Source: CAD feature listing. Evaluate the final solid. Frame: model axes, mm. A direction names the side the tool comes from. Give positions to 0.01 mm unless a question says otherwise; leave off trailing zeros. Write each loop counter-clockwise with the first axis right and the second up, starting at its lowest first coordinate (ties: lowest second). Pieces come first, ordered by that corner, then holes. Notation, with made-up numbers: (75.25, 50.5) -> (97.25, 50.5) arc R15 ccw to (97.25, 63.5) -> close; hole circle Ø7 at (1, -38). An arc over 180 degrees is marked (long way). Write item = value, one per line.
from build123d import *

# Parameters (mm, degrees)
F0_W     = 42.3
F0_H     = 42.3
F1_DEPTH = 21.15
F2_SIZE  = 5
F3_R     = 11
F4_DEPTH = 2
F5_R     = 2.5
F6_DEPTH = 22


with BuildPart() as f1:
    # F0 (on Front) → F1 (new body, symmetric)
    with BuildSketch(Plane.XZ):
        Rectangle(F0_W, F0_H)
    extrude(amount=F1_DEPTH, both=True)

    # F2
    f2_edges = [f1.edges().sort_by_distance(p)[0] for p in [
        (-21.15, 0, 21.15),
        (21.15, 0, 21.15),
        (-21.15, 0, -21.15),
        (21.15, 0, -21.15),
    ]]
    chamfer(f2_edges, length=F2_SIZE)

    # F3 (on face) → F4 (join)
    with BuildSketch(Plane.XZ.offset(21.15)):
        Circle(F3_R)
    extrude(amount=F4_DEPTH)

    # F5 (on face) → F6 (join)
    with BuildSketch(Plane.XZ.offset(23.15)):
        Circle(F5_R)
    extrude(amount=F6_DEPTH)


solid = f1.part
(1) Section query A-A (y = 11). Return loops of the section in (x, z), plus the area to 3 significant figures.
Values follow:
outline = (-21.15, -16.15) -> (-16.15, -21.15) -> (16.15, -21.15) -> (21.15, -16.15) -> (21.15, 16.15) -> (16.15, 21.15) -> (-16.15, 21.15) -> (-21.15, 16.15) -> close
area = 1,740 mm2
(2) Section query C-C (z = 0). Return loops of the section in (x, y), plus the area to 3 significant figures.
Values follow:
outline = (-21.15, -21.15) -> (-11, -21.15) -> (-11, -23.15) -> (-2.5, -23.15) -> (-2.5, -45.15) -> (2.5, -45.15) -> (2.5, -23.15) -> (11, -23.15) -> (11, -21.15) -> (21.15, -21.15) -> (21.15, 21.15) -> (-21.15, 21.15) -> close
area = 1,940 mm2
(3) Material intervals for line 1 (Y direction, x = 11.5, z = -12.5); line 2 (Y direction, x = 0, z = -8); line 3 (Z direction, x = -18.5, y = 1), sorted ascending.
Values follow:
line_1 = -21.15 to 21.15
line_2 = -23.15 to 21.15
line_3 = -18.8 to 18.8
(4) First-contact query: pin 1 (3 mm diameter, centred on x = -6.5, z = 15, fed in from -Y); pin 2 (3 mm diameter, centred on x = 4.5, z = 6.5, fed in from -Y). Flat tips, straight axial feed; report the tip coordinate or a pass-through.
Values follow:
pin_1 = -21.15
pin_2 = -23.15
(5) Section query D-D (x = 8). Return loops of the section in (y, z).
Values follow:
outline = (-23.15, -7.55) -> (-21.15, -7.55) -> (-21.15, -21.15) -> (21.15, -21.15) -> (21.15, 21.15) -> (-21.15, 21.15) -> (-21.15, 7.55) -> (-23.15, 7.55) -> close
(6) Access query for faces 1 (the face through (-2.38, -22.14, -10.74)), 2 (the face through (0, -45.15, 0)). Directions: +Z, -Z, +X, -X, +Y, -Y. A direction counts if a zero-diameter tool reaches every point of the face in a straight line with its end or side. Return the directions, or none.
Values follow:
face_1 = -Y
face_2 = +Z, -Z, +X, -X, -Y
(7) Section query B-B (x = 0). Return loops of the section in (y, z).
Values follow:
outline = (-45.15, -2.5) -> (-23.15, -2.5) -> (-23.15, -11) -> (-21.15, -11) -> (-21.15, -21.15) -> (21.15, -21.15) -> (21.15, 21.15) -> (-21.15, 21.15) -> (-21.15, 11) -> (-23.15, 11) -> (-23.15, 2.5) -> (-45.15, 2.5) -> close
